The model under review builds one solid part; all positions refer to its coordinate system, in mm. Coordinates: 2 decimals unless noted, no trailing zeros. Loops run counter-clockwise (first coordinate to the right, second up) from the corner with the lowest first, then second, coordinate; pieces in that order, holes last. Notation, with made-up numbers: (58, -17) - (89, -17) arc R10 cw to (89, -1) - close; hole circle Ø6 at (-5, -36.5). An arc over 180 degrees is marked (long way). One line per item, written item: value. Start each with the question number.
1. We need section A-A, the plane z = 29.5. Give the boundary of the cut face in (x, y).
2. We need section D-D, the plane z = 25.5. Give the boundary of the cut face in (x, y), then the cut area to 3 significant figures.
3. To check wall thickness, follow line 1 (X direction, y = -0.2, z = 35.25); line 2 (X direction, y = -0.4, z = 34.75); line 3 (X direction, y = -0.7, z = 21). State the ranges of each line that lie inside material, in increasing order.
4. We need section C-C, the plane y = -0.8. Give the boundary of the cut face in (x, z).
5. We need section B-B, the plane x = 91. Give the boundary of the cut face in (y, z), then the cut area to 3 significant figures.
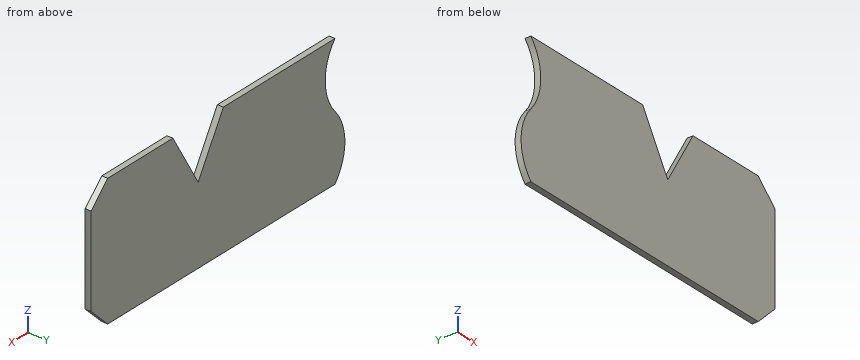
from build123d import *

# Parameters (mm, degrees)
F1_DEPTH = 1


with BuildPart() as f1:
    # F0 (on Front) → F1 (new body)
    with BuildSketch(Plane.XZ):
        with BuildLine():
            Line((113.174544, 36.973573), (90.174544, 36.973573))
            ThreePointArc((90.174544, 36.973573), (92.196906, 31.473573), (90.174544, 25.973573))
            ThreePointArc((90.174544, 25.973573), (88.152182, 20.473573), (90.174544, 14.973573))
            Line((90.174544, 14.973573), (111.174544, 14.973573))
            Line((111.174544, 14.973573), (121.566849, 14.973573))
            Line((121.566849, 14.973573), (136.993918, 14.973573))
            Line((136.993918, 14.973573), (140.403688, 18.383343))
            Line((140.403688, 18.383343), (140.403688, 25.973573))
            Line((140.403688, 25.973573), (140.403688, 33.563804))
            Line((140.403688, 33.563804), (136.993918, 36.973573))
            Line((136.993918, 36.973573), (123.566849, 36.973573))
            Line((123.566849, 36.973573), (118.370696, 27.973573))
            Line((118.370696, 27.973573), (113.174544, 36.973573))
        make_face()
    extrude(amount=F1_DEPTH)


solid = f1.part
Findings below:
1. outline: (91.96, -1) - (117.49, -1) - (117.49, 0) - (91.96, 0) - close; (119.25, -1) - (140.4, -1) - (140.4, 0) - (119.25, 0) - close
2. outline: (89.8, -1) - (140.4, -1) - (140.4, 0) - (89.8, 0) - close
2. area: 50.6 mm2
3. line 1: 91.31 to 114.17, 122.57 to 138.72
3. line 2: 91.54 to 114.46, 122.28 to 139.22
3. line 3: 88.17 to 140.4
4. outline: (90.17, 14.97) - (136.99, 14.97) - (140.4, 18.38) - (140.4, 33.56) - (136.99, 36.97) - (123.57, 36.97) - (118.37, 27.97) - (113.17, 36.97) - (90.17, 36.97) arc R8.49 cw to (90.17, 25.97) arc R8.49 ccw to start
5. outline: (-1, 14.97) - (0, 14.97) - (0, 27.13) - (-1, 27.13) - close; (-1, 35.82) - (0, 35.82) - (0, 36.97) - (-1, 36.97) - close
5. area: 13.3 mm2
